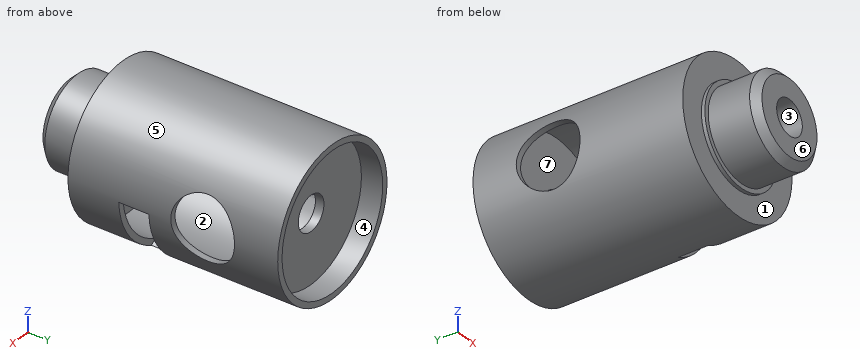
Autodesk Inventor part; units mm, degrees
ref_plane "YZ Plane" through (0, 0, 0) normal (1, 0, 0) x (0, 1, 0)
ref_plane "XZ Plane" through (0, 0, 0) normal (0, 1, 0) x (-1, 0, 0)
ref_plane "XY Plane" through (0, 0, 0) normal (0, 0, 1) x (1, 0, 0)
sketch "Sketch1" plane through (0, 0, 0) normal (0, 1, 0) x (-1, 0, 0)
  circle A0 centre (0, 0) radius 5.2959
  dimension "d0" = 10.5918
extrude "Extrusion1" add sketch "Sketch1" along normal blind 15.0368
sketch "Sketch3" plane through (0, 15.0368, 0) normal (0, 1, 0) x (1, 0, 0)
  circle A0 centre (0, 0) radius 3.4925
  dimension "d6" = 6.985
extrude "Extrusion3" add sketch "Sketch3" against normal blind 15.2908
sketch "Sketch4" plane through (0, 15.0368, 0) normal (0, 1, 0) x (1, 0, 0)
  circle A0 centre (0, 0) radius 3.175
  dimension "d9" = 6.35
extrude "Extrusion4" add sketch "Sketch4" against normal blind 18.7706
sketch "Sketch9" plane through (0, -3.7338, 0) normal (0, -1, 0) x (1, 0, 0)
  circle A0 centre (0, 0) radius 5.2959
hole "Hole1" at (0, -3.7338, 0) direction (0, 1, 0) diameter 2.4892 end through all
sketch "Sketch10" plane through (0, 0, 0) normal (1, 0, 0) x (0, 1, 0)
  line L0 (15.0368, -5.2959) -> (15.0368, 5.2959)
  line L1 (15.0368, -5.256) -> (9.6521, -5.2959)
  line L2 (0, -5.2959) -> (15.0368, -5.2959)
  circle A0 centre (9.6521, 0) radius 2.286
  point P0 (0, 0)
  dimension "d33" = 5.3848
  dimension "d34" = 4.572
extrude "Extrusion7" cut sketch "Sketch10" along normal mid plane 12.446 contours A0
sketch "Sketch5" plane through (0, 15.0368, 0) normal (0, 1, 0) x (1, 0, 0)
  circle A0 centre (0, 0) radius 4.8768
  dimension "d12" = 9.7536
extrude "Extrusion5" cut sketch "Sketch5" against normal blind 1.524
ref_plane "Work Plane3" through (0, 12.9032, 0) normal (0, 1, 0) x (-1, 0, 0)
sketch "Sketch8" plane through (0, 12.9032, 0) normal (0, 1, 0) x (-1, 0, 0)
  circle A0 centre (0, 0) radius 4.8768
extrude "Extrusion6" cut sketch "Sketch8" against normal blind 12.446
ref_plane "Work Plane4" through (0, 3.6322, 0) normal (0, -1, 0) x (1, 0, 0)
chamfer "Chamfer1" distance 0.508 angle 45 1 edges at (-3.175, -3.7338, 0)
sketch "Sketch11" plane through (0, 3.6322, 0) normal (0, -1, 0) x (1, 0, 0)
  circle A0 centre (0, 0) radius 5.2959
  circle A1 centre (0, 0) radius 4.8768
  line L0 (4.8768, 0) -> (1.7044, -4.5693)
  line L1 (2.1158, -4.8549) -> (5.2959, -0.291)
  line L2 (4.8768, 0) -> (5.9401, -0.7399)
  line L3 (5.9401, -0.7399) -> (2.763, -5.3059)
  line L4 (2.763, -5.3059) -> (1.7044, -4.5693)
  dimension "d37" = 5.5626
  dimension "d38" = 1.2954
extrude "Extrusion8" cut sketch "Sketch11" against normal blind 2.159 contours L1 A1 A0 | L4 A1 L1 | A0 L1 L2 L3 L4 | L2 L1 A0 | A0 L1 A1 L2 | L1 A1 | A1 L0 L1 | A1 L0
thread "Thread1"
properties part number "Mixture  Control"
Geometry check sheet. Reference: the model listing, model coordinates, mm. Face numbers are marked on the shaded views. A direction names the side the tool comes from. Round coordinates to 2 decimals unless told otherwise and drop trailing zeros. Write each loop counter-clockwise with the first axis right and the second up, starting at its lowest first coordinate (ties: lowest second). Pieces come first, ordered by that corner, then holes. Notation, with made-up numbers: (13, 18) -> (52, 18) arc R25 ccw to (52, 31) -> close; hole circle Ø5 at (84.25, 59). An arc over 180 degrees is marked (long way). One line per item, written item: value. Start each with the question number.
(1) Scan lines: line 1 (Z direction, x = 0, y = 9.75); line 2 (Y direction, x = -2.5, z = 2.75); line 3 (Y direction, x = 2.5, z = -4.5). Record each from-to range of solid material in increasing order. Write a range as [from, to].
(2) Cross-section at C-C, the plane y = -0.75. Record the cut outline in (x, z) (3 decimals).
(3) Cross-section at D-D, the plane z = 0.5. Give the number of separate pieces and of enclosed holes in the cut face, and give its area (3 significant figures).
(4) Go/stop test with flat-tipped pins: pin 1 Ø3 at (x, z) = (-2.5, 2) entering from +Y; pin 2 Ø1.1 at (x, z) = (4, -2) entering from -Y; pin 3 Ø2 at (y, z) = (-1.5, 3.5) entering from +X. Record where each tip stops, or that it passes through.
(5) Draft check along Z on the marked faces 5, 6 and 7. Enter one of: +Z half, -Z half, draft (parallel to the pull), parting line (faces both ways), or undercut.
(6) Access from +Z, -Z, +X, -X, +Y, -Y to the whole of each face (thin tool, end or side, straight path). Record for the marked faces 1, 2, 3 and 4.
(7) Cross-section at B-B, the plane y = 9.5. Record the cut outline in (x, z), and give its area (3 significant figures).
Answer:
1. line 1: [-5.3, -4.88], [4.88, 5.3]
1. line 2: [0, 0.46], [12.9, 13.51]
1. line 3: [0, 3.63], [5.79, 15.04]
2. outline: circle Ø6.35 at (0, 0); hole circle Ø2.489 at (0, 0)
3. separate pieces: 4
3. enclosed holes: 0
3. area: 31.6 mm²
4. pin 1: y = 13.51
4. pin 2: y = 0
4. pin 3: x = 1.96
5. face 5: parting line
5. face 6: draft
5. face 7: undercut
6. face 1: -Y
6. face 2: none
6. face 3: +Y, -Y
6. face 4: +Y
7. outline: (-4.78, -2.28) arc R5.3 ccw to (4.78, -2.28) -> (4.31, -2.28) arc R4.88 cw to (-4.31, -2.28) -> close; (-4.78, 2.28) -> (-4.31, 2.28) arc R4.88 cw to (4.31, 2.28) -> (4.78, 2.28) arc R5.3 ccw to start
7. area: 9.43 mm²
